```python
from build123d import *

# Parameters (mm, degrees)
BOSS_EXTRUDE1_DEPTH             = 6.8
BOSS_EXTRUDE2_REACH             = 10.744
SKETCH2_W                       = 0.335114676
SKETCH2_H                       = 0.8
BOSS_EXTRUDE2_DIRECTION_2_DEPTH = 1
SKETCH3_W                       = 5.5
SKETCH3_H                       = 0.5
CUT_EXTRUDE1_DEPTH              = 5


with BuildPart() as part:
    # Sketch1 → Boss-Extrude1 (new body)
    with BuildSketch(Plane.XY):
        with BuildLine():
            Line((-2.97, 1.6), (2.97, 1.6))
            ThreePointArc((2.97, 1.6), (4.030660172, 1.160660172), (4.47, 0.1))
            Line((4.47, 0.1), (4.47, -0.1))
            ThreePointArc((4.47, -0.1), (4.030660172, -1.160660172), (2.97, -1.6))
            Line((2.97, -1.6), (-2.97, -1.6))
            ThreePointArc((-2.97, -1.6), (-4.030660172, -1.160660172), (-4.47, -0.1))
            Line((-4.47, -0.1), (-4.47, 0.1))
            ThreePointArc((-4.47, 0.1), (-4.030660172, 1.160660172), (-2.97, 1.6))
        make_face()
    extrude(amount=BOSS_EXTRUDE1_DEPTH)

    # Sketch2 → Boss-Extrude2 (add, up to next)
    with BuildSketch(Plane.XZ.offset(1.6), mode=Mode.PRIVATE) as boss_extrude2_sk1:
        with Locations((-4.302442662, 4.2)):
            Rectangle(SKETCH2_W, SKETCH2_H)
    boss_extrude2_tool1 = extrude(boss_extrude2_sk1.sketch, amount=-BOSS_EXTRUDE2_REACH, mode=Mode.PRIVATE) - part.part
    # Sketch2 → Boss-Extrude2 (add, up to next)
    with BuildSketch(Plane.XZ.offset(1.6), mode=Mode.PRIVATE) as boss_extrude2_sk2:
        with Locations((-4.302442662, 0.4)):
            Rectangle(SKETCH2_W, SKETCH2_H)
    boss_extrude2_tool2 = extrude(boss_extrude2_sk2.sketch, amount=-BOSS_EXTRUDE2_REACH, mode=Mode.PRIVATE) - part.part
    # Sketch2 → Boss-Extrude2 (add, up to next)
    with BuildSketch(Plane.XZ.offset(1.6), mode=Mode.PRIVATE) as boss_extrude2_sk3:
        with Locations((4.302442662, 0.4)):
            Rectangle(SKETCH2_W, SKETCH2_H)
    boss_extrude2_tool3 = extrude(boss_extrude2_sk3.sketch, amount=-BOSS_EXTRUDE2_REACH, mode=Mode.PRIVATE) - part.part
    # Sketch2 → Boss-Extrude2 (add, up to next)
    with BuildSketch(Plane.XZ.offset(1.6), mode=Mode.PRIVATE) as boss_extrude2_sk4:
        with Locations((4.302442662, 4.2)):
            Rectangle(SKETCH2_W, SKETCH2_H)
    boss_extrude2_tool4 = extrude(boss_extrude2_sk4.sketch, amount=-BOSS_EXTRUDE2_REACH, mode=Mode.PRIVATE) - part.part
    add(boss_extrude2_tool1.solids().sort_by_distance((-4.302443, -1.6, 4.2))[0])
    add(boss_extrude2_tool2.solids().sort_by_distance((-4.302443, -1.6, 0.4))[0])
    add(boss_extrude2_tool3.solids().sort_by_distance((4.302443, -1.6, 0.4))[0])
    add(boss_extrude2_tool4.solids().sort_by_distance((4.302443, -1.6, 4.2))[0])

    # Sketch2 → Boss-Extrude2 direction 2 (add)
    with BuildSketch(Plane.XZ.offset(1.6)):
        with Locations((-4.302442662, 4.2)):
            Rectangle(SKETCH2_W, SKETCH2_H)
        with Locations((-4.302442662, 0.4)):
            Rectangle(SKETCH2_W, SKETCH2_H)
        with Locations((4.302442662, 0.4)):
            Rectangle(SKETCH2_W, SKETCH2_H)
        with Locations((4.302442662, 4.2)):
            Rectangle(SKETCH2_W, SKETCH2_H)
    extrude(amount=BOSS_EXTRUDE2_DIRECTION_2_DEPTH)

    # Sketch3 → Cut-Extrude1 (cut)
    with BuildSketch(Plane.XY.offset(6.8)):
        with BuildLine():
            Line((-2.97, -1.4), (2.97, -1.4))
            ThreePointArc((2.97, -1.4), (3.889238816, -1.019238816), (4.27, -0.1))
            Line((4.27, -0.1), (4.27, 0.1))
            ThreePointArc((4.27, 0.1), (3.889238816, 1.019238816), (2.97, 1.4))
            Line((2.97, 1.4), (-2.97, 1.4))
            ThreePointArc((-2.97, 1.4), (-3.889238816, 1.019238816), (-4.27, 0.1))
            Line((-4.27, 0.1), (-4.27, -0.1))
            ThreePointArc((-4.27, -0.1), (-3.889238816, -1.019238816), (-2.97, -1.4))
        make_face()
        Rectangle(SKETCH3_W, SKETCH3_H, mode=Mode.SUBTRACT)
    extrude(amount=-CUT_EXTRUDE1_DEPTH, mode=Mode.SUBTRACT)


solid = part.part
```
Model file for the job. Use its own axes, mm. A direction names the side the tool comes from. Coordinates: 2 decimals unless noted, no trailing zeros. Order: outer loops, then holes, each group sorted by start corner. A loop starts at its lowest first (then second) coordinate and runs counter-clockwise, first axis right, second up. Notation, with made-up numbers: (-0.75, 58.5) - (22.25, 58.5) arc R34 cw to (22.25, 89.5) - close; hole circle Ø6 at (55, 74.25). An arc over 180 degrees is marked (long way). Return JSON: item names as keys, results as strings. Group by question number.
1) Saw through at B-B, the plane y = -1.3. Write the cut outline in (x, z), plus the area to 3 significant figures.
2) Saw through at C-C, the plane y = -2.05. Write the cut outline in (x, z).
3) Mould opens along Y. For faces 1 (the cylindrical face through (3.88, -1.03, 4.34)), 2 (the flat face through (4.135, -2, 4)), 3 (the cylindrical face through (4.02, 1.17, 3.35)) say: released by +Y, released by -Y, zero draft, split by the parting line, or undercut.
4) Flat gauge pins, fed straight in: P1, Ø2.5, axis at x = 0.5, z = 5, coming from the -Y side; P2, Ø1.4, axis at x = -2, y = 0.5, coming from the +Z side. Where does each tip first touch, or does it go through?
5) Probe line 1 (Y direction, x = 2, z = 4.25); line 2 (X direction, y = -0.15, z = 4); line 3 (Z direction, x = 3.5, y = -0.4). List the from-to ranges inside material, lowest first. Write a range as from..to.
6) Saw through at A-A, the plane z = 2.75. Write the cut outline in (x, y), plus the area to 3 significant figures.
7) Tool access for faces 4 (the flat face through (0, 1.4, 4)), 5 (the cylindrical face through (-4.04, 1.15, 3.35)), 6 (the flat face through (-4.135, -2, 4)): list every direction of +Z, -Z, +X, -X, +Y, -Y with a clear straight run to the whole face (end or side of a thin tool).
8) Saw through at D-D, the plane z = 4.5. Write the cut outline in (x, y) (3 decimals).
Values found:
{
 "1": {"outline": "(-4.47, 0) - (-4.13, 0) - (-4.13, 0.8) - (-4.47, 0.8) - close; (-4.47, 3.8) - (-4.13, 3.8) - (-4.13, 4.6) - (-4.47, 4.6) - close; (-3.87, 0) - (3.87, 0) - (3.87, 6.8) - (3.47, 6.8) - (3.47, 1.8) - (-3.47, 1.8) - (-3.47, 6.8) - (-3.87, 6.8) - close; (4.13, 0) - (4.47, 0) - (4.47, 0.8) - (4.13, 0.8) - close; (4.13, 3.8) - (4.47, 3.8) - (4.47, 4.6) - (4.13, 4.6) - close", "area": "19.0 mm²"},
 "2": {"outline": "(-4.47, 0) - (-4.13, 0) - (-4.13, 0.8) - (-4.47, 0.8) - close; (-4.47, 3.8) - (-4.13, 3.8) - (-4.13, 4.6) - (-4.47, 4.6) - close; (4.13, 0) - (4.47, 0) - (4.47, 0.8) - (4.13, 0.8) - close; (4.13, 3.8) - (4.47, 3.8) - (4.47, 4.6) - (4.13, 4.6) - close"},
 "3": {"face 1": "undercut", "face 2": "zero draft", "face 3": "released by +Y"},
 "4": {"P1": "stops at y = -1.6", "P2": "stops at z = 6.8"},
 "5": {"line 1": "y = -1.6..-1.4, -0.25..0.25, 1.4..1.6", "line 2": "x = -4.47..-4.27, -2.75..2.75, 4.27..4.47", "line 3": "z = 0..1.8"},
 "6": {"outline": "(-4.47, -0.1) arc R1.5 ccw to (-2.97, -1.6) - (2.97, -1.6) arc R1.5 ccw to (4.47, -0.1) - (4.47, 0.1) arc R1.5 ccw to (2.97, 1.6) - (-2.97, 1.6) arc R1.5 ccw to (-4.47, 0.1) - close; (-2.75, -0.25) - (2.75, -0.25) - (2.75, 0.25) - (-2.75, 0.25) - close; hole (-4.27, -0.1) arc R1.3 ccw to (-2.97, -1.4) - (2.97, -1.4) arc R1.3 ccw to (4.27, -0.1) - (4.27, 0.1) arc R1.3 ccw to (2.97, 1.4) - (-2.97, 1.4) arc R1.3 ccw to (-4.27, 0.1) - close", "area": "6.97 mm²"},
 "7": {"face 4": "+Z", "face 5": "+Z, -Z, -X, +Y", "face 6": "+Z, -Z, -Y"},
 "8": {"outline": "(-4.47, -2.6) - (-4.135, -2.6) - (-4.135, -1.045) arc R1.5 ccw to (-2.97, -1.6) - (2.97, -1.6) arc R1.5 ccw to (4.135, -1.045) - (4.135, -2.6) - (4.47, -2.6) - (4.47, 0.1) arc R1.5 ccw to (2.97, 1.6) - (-2.97, 1.6) arc R1.5 ccw to (-4.47, 0.1) - close; (-2.75, -0.25) - (2.75, -0.25) - (2.75, 0.25) - (-2.75, 0.25) - close; hole (-4.27, -0.1) arc R1.3 ccw to (-2.97, -1.4) - (2.97, -1.4) arc R1.3 ccw to (4.27, -0.1) - (4.27, 0.1) arc R1.3 ccw to (2.97, 1.4) - (-2.97, 1.4) arc R1.3 ccw to (-4.27, 0.1) - close"}
}
